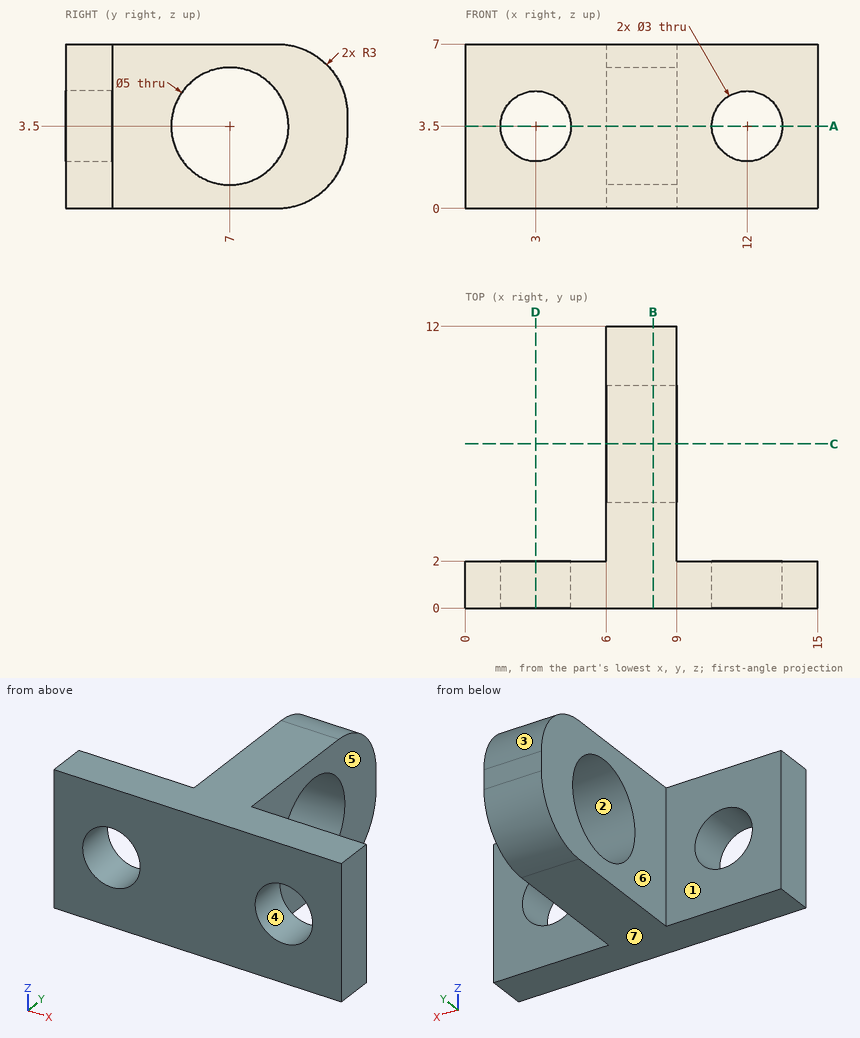
The drawing under review shows one solid part. Ordinate dimensions are in mm from its lowest x, y, z. A direction names the side the tool comes from. Give positions to 0.01 mm unless a question says otherwise; leave off trailing zeros. Order: outer loops, then holes, each group sorted by start corner. A loop starts at its lowest first (then second) coordinate and runs counter-clockwise, first axis right, second up. Notation, with made-up numbers: (68, -31) - (126, -31) arc R17 cw to (126, -20) - close; hole circle Ø9 at (-18.5, 24). An arc over 180 degrees is marked (long way). Answer as a JSON object with one key per item and string values. Group by question number.
Item 1: Take a section at A-A on z = 3.5. Give the boundary of the cut face in (x, y).
Item 2: Clearance check with flat-ended pins moving along their axes: pin 1 Ø4 at (y, z) = (3.5, 0.5) entering from -X; pin 2 Ø1.8 at (x, z) = (3, 3.5) entering from -Y; pin 3 Ø1.8 at (x, z) = (2, 5) entering from +Y. State where each tip first meets the part, or that it passes through.
Item 3: Draft analysis for pull direction Z (two halves, no side actions). For the marked faces 1, 2, 3 and 4, state which applies: pulls with the +Z half, pulls with the -Z half, needs draft (parallel to the pull), parting line crosses it, or undercut.
Item 4: Take a section at B-B on x = 8. Give the boundary of the cut face in (y, z).
Item 5: Wall thickness on line 1 along X through (y, z) = (0.5, 3.5); line 2 along Y through (x, z) = (6.5, 3.5); line 3 along X through (y, z) = (1.25, 2.75): over which ranges is each line inside the solid? List them lowest first.
Item 6: Take a section at D-D on x = 3. Give the boundary of the cut face in (y, z).
Item 7: Take a section at C-C on y = 7. Give the boundary of the cut face in (x, z), and give its area (3 significant figures).
Item 8: Machinability: for the marked faces 5, 6 and 7, which of the approach directions +Z, -Z, +X, -X, +Y, -Y give a long, thin tool a straight path to every point of the face, cutting with its end or side? Answer none if there is none.
Reported:
{
 "1": {"outline": "(0, 0) - (1.5, 0) - (1.5, 2) - (0, 2) - close; (4.5, 0) - (10.5, 0) - (10.5, 2) - (9, 2) - (9, 4.5) - (6, 4.5) - (6, 2) - (4.5, 2) - close; (6, 9.5) - (9, 9.5) - (9, 12) - (6, 12) - close; (13.5, 0) - (15, 0) - (15, 2) - (13.5, 2) - close"},
 "2": {"pin 1": "x = 0", "pin 2": "through", "pin 3": "y = 2"},
 "3": {"face 1": "needs draft", "face 2": "undercut", "face 3": "pulls with the +Z half", "face 4": "undercut"},
 "4": {"outline": "(0, 0) - (9, 0) arc R3 ccw to (12, 3) - (12, 4) arc R3 ccw to (9, 7) - (0, 7) - close; hole circle Ø5 at (7, 3.5)"},
 "5": {"line 1": "0 to 1.5, 4.5 to 10.5, 13.5 to 15", "line 2": "0 to 4.5, 9.5 to 12", "line 3": "0 to 1.7, 4.3 to 10.7, 13.3 to 15"},
 "6": {"outline": "(0, 0) - (2, 0) - (2, 2) - (0, 2) - close; (0, 5) - (2, 5) - (2, 7) - (0, 7) - close"},
 "7": {"outline": "(6, 0) - (9, 0) - (9, 1) - (6, 1) - close; (6, 6) - (9, 6) - (9, 7) - (6, 7) - close", "area": "6.00 mm^2"},
 "8": {"face 5": "+Z, -Z, +X, +Y", "face 6": "+Z, -Z, -X, +Y", "face 7": "-Z, +X, -X, +Y, -Y"}
}
